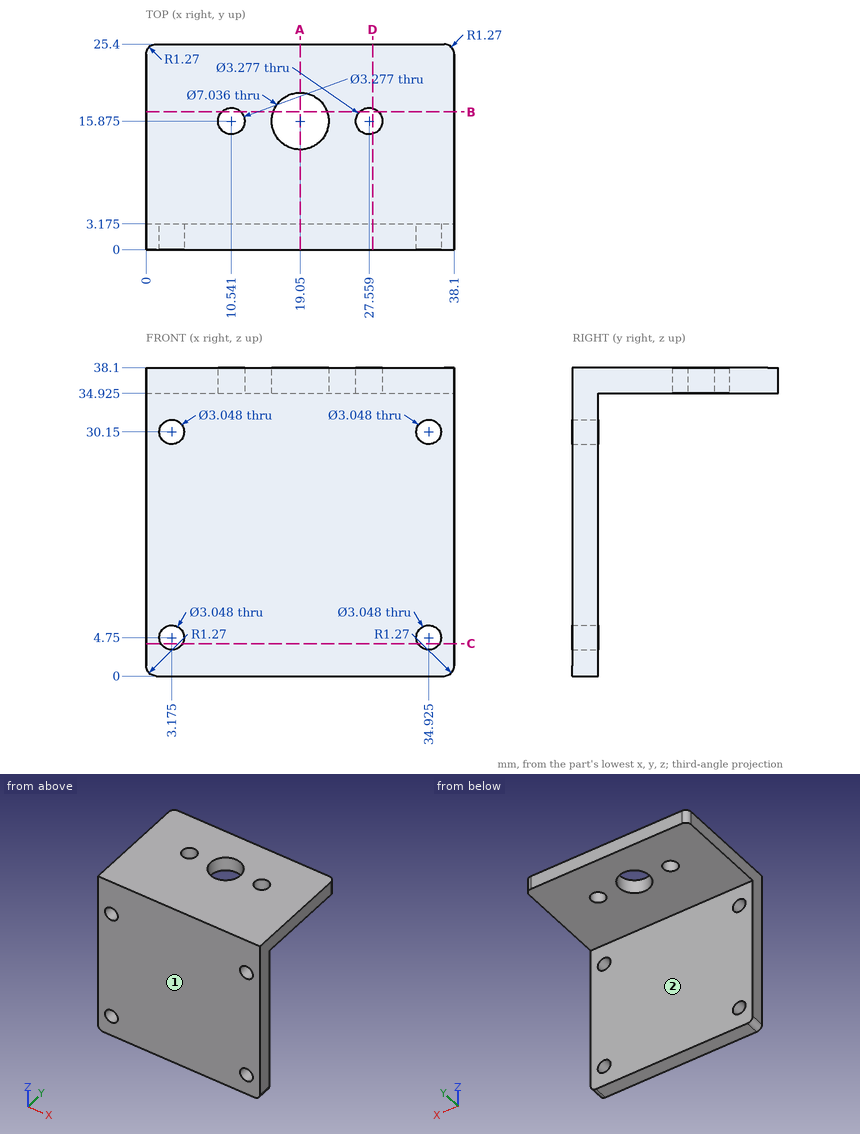
Check sheet for the drawn part. Datum: minimum x, y, z corner. Units: mm. A direction names the side the tool comes from. Round coordinates to 2 decimals unless told otherwise and drop trailing zeros. Loops run counter-clockwise (first coordinate to the right, second up) from the corner with the lowest first, then second, coordinate; pieces in that order, holes last. Notation, with made-up numbers: (29, -16) - (73, -16) arc R9 ccw to (73, -12) - close; hole circle Ø2 at (52.5, 52). An arc over 180 degrees is marked (long way). Use one line per item in the form item = value.
1. Section check B-B on y = 17. Give the number of separate pieces and of enclosed holes in the cut face.
A:
separate_pieces = 4
enclosed_holes = 0
2. Scan lines: probe 1 along Z at (x, y) = (2.5, 2) (1 decimal); probe 2 along Z at (x, y) = (35, 21.25) (1 decimal); probe 3 along Y at (x, z) = (34, 16.5) (1 decimal). Record each from-to range of solid material in increasing order.
A:
probe_1 = 0 to 3.4, 6.1 to 28.8, 31.5 to 38.1
probe_2 = 34.9 to 38.1
probe_3 = 0 to 3.2
3. Section check A-A on x = 19.05. Record the cut outline in (y, z) (1 decimal), and give its area (3 significant figures).
A:
outline = (0, 0) - (3.2, 0) - (3.2, 34.9) - (12.4, 34.9) - (12.4, 38.1) - (0, 38.1) - close; (19.4, 34.9) - (25.4, 34.9) - (25.4, 38.1) - (19.4, 38.1) - close
area = 169 mm²
4. Access from +Z, -Z, +X, -X, +Y, -Y to the whole of each face (thin tool, end or side, straight path). Record for the marked faces 1 and 2.
A:
face_1 = +Z, -Z, +X, -X, -Y
face_2 = -Z, +X, -X, +Y
5. Section check D-D on x = 28. Record the cut outline in (y, z) (1 decimal).
A:
outline = (0, 0) - (3.2, 0) - (3.2, 34.9) - (14.3, 34.9) - (14.3, 38.1) - (0, 38.1) - close; (17.5, 34.9) - (25.4, 34.9) - (25.4, 38.1) - (17.5, 38.1) - close
6. Gauge pin test, flat ends, axial feed: pin 1 Ø1.5 at (x, z) = (24.5, 6) entering from +Y (3 decimals); pin 2 Ø9 at (x, y) = (19.05, 15.875) entering from +Z; pin 3 Ø5 at (x, y) = (27.559, 15.875) entering from -Z (3 decimals). Record the tip position at first contact, or that the pin passes through.
A:
pin_1 = 3.175
pin_2 = 38.1
pin_3 = 34.925
7. Section check C-C on z = 4. Record the cut outline in (x, y) (1 decimal).
A:
outline = (0, 0) - (1.8, 0) - (1.8, 3.2) - (0, 3.2) - close; (4.5, 0) - (33.6, 0) - (33.6, 3.2) - (4.5, 3.2) - close; (36.3, 0) - (38.1, 0) - (38.1, 3.2) - (36.3, 3.2) - close
